```python
from build123d import *

# Parameters (mm, degrees)
SKETCH2_R          = 1.9177
CUT_EXTRUDE1_DEPTH = 33.764861657


with BuildPart() as part:
    # Sketch1 → Revolve1 (revolve)
    with BuildSketch(Plane.XY, mode=Mode.PRIVATE) as revolve1_sk:
        with BuildLine():
            Line((0, 0), (0, 30.1625))
            Line((0, 30.1625), (4.953, 30.1625))
            Line((4.953, 30.1625), (5.588, 20.76733075))
            Line((5.588, 20.76733075), (6.904482, 20.76733075))
            Line((6.904482, 20.76733075), (7.04215, 19.64973075))
            ThreePointArc((7.04215, 19.64973075), (4.64185, 17.316376969), (7.183974364, 15.1384))
            Line((7.183974364, 15.1384), (7.321642364, 14.0208))
            Line((7.321642364, 14.0208), (4.622892364, 14.0208))
            Line((4.622892364, 14.0208), (4.773075636, 12.8016))
            Line((4.773075636, 12.8016), (7.471825636, 12.8016))
            Line((7.471825636, 12.8016), (7.609493636, 11.684))
            Line((7.609493636, 11.684), (4.910743636, 11.684))
            Line((4.910743636, 11.684), (5.060926909, 10.4648))
            Line((5.060926909, 10.4648), (7.759676909, 10.4648))
            Line((7.759676909, 10.4648), (7.897344909, 9.3472))
            Line((7.897344909, 9.3472), (5.198594909, 9.3472))
            Line((5.198594909, 9.3472), (5.348778182, 8.128))
            Line((5.348778182, 8.128), (8.047528182, 8.128))
            Line((8.047528182, 8.128), (8.185196182, 7.0104))
            Line((8.185196182, 7.0104), (5.486446182, 7.0104))
            Line((5.486446182, 7.0104), (5.636629455, 5.7912))
            Line((5.636629455, 5.7912), (8.335379455, 5.7912))
            Line((8.335379455, 5.7912), (8.473047455, 4.6736))
            Line((8.473047455, 4.6736), (5.774297455, 4.6736))
            Line((5.774297455, 4.6736), (5.924480727, 3.4544))
            Line((5.924480727, 3.4544), (8.623230727, 3.4544))
            Line((8.623230727, 3.4544), (8.760898727, 2.3368))
            Line((8.760898727, 2.3368), (6.062148727, 2.3368))
            Line((6.062148727, 2.3368), (6.212332, 1.1176))
            Line((6.212332, 1.1176), (8.911082, 1.1176))
            Line((8.911082, 1.1176), (9.04875, 0))
            Line((9.04875, 0), (0, 0))
        make_face()
    revolve(revolve1_sk.sketch.rotate(Axis((0, 0, 0), (0, 1, 0)), 90), axis=Axis((0, 0, 0), (0, 1, 0)))

    # Sketch2 → Cut-Extrude1 (cut, through all)
    with BuildSketch(Plane(origin=(0, 30.1625, 0), x_dir=(1, 0, 0), z_dir=(0, 1, 0))):
        with Locations(Location((0, 0, 0), (0, 0, 270))):
            Circle(SKETCH2_R)
    extrude(amount=-CUT_EXTRUDE1_DEPTH, mode=Mode.SUBTRACT)


solid = part.part
```
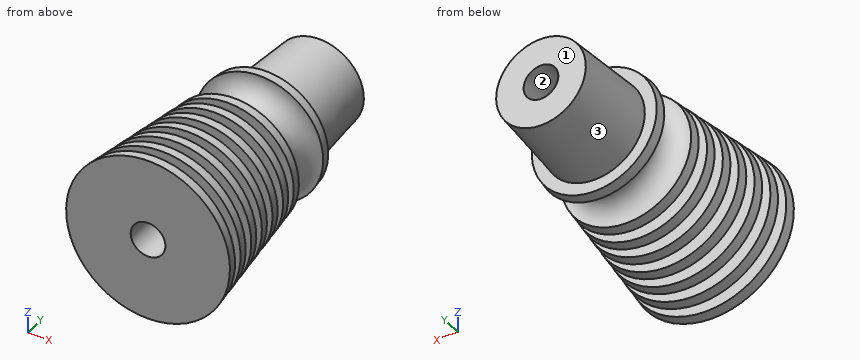
Design review of the part built by this model. Coordinates are the model's own, in mm. Face numbers are marked on the shaded views. Round coordinates to 2 decimals unless told otherwise and drop trailing zeros. Write each loop counter-clockwise with the first axis right and the second up, starting at its lowest first coordinate (ties: lowest second). Pieces come first, ordered by that corner, then holes.
Item 1: The part is to be moulded in two halves that separate along Z. For the marked faces 1, 2 and 3, say which applies: +Z half, -Z half, draft (parallel to the pull), parting line (faces both ways), or undercut.
Item 2: For probe 1 along X at (y, z) = (20.5, -1.75); probe 2 along X at (y, z) = (11, 0) (3 decimals); probe 3 along X at (y, z) = (9.5, 2.5), list the stretches that pass through material, from the lowest coordinate up.
Item 3: We need section A-A on y = 7.5. Write out the cut boundary in (x, z), and give its area (3 significant figures).
Item 4: Clearance check with flat-ended pins moving along their axes: pin 1 Ø3 at (x, z) = (-5, 1) entering from -Y; pin 2 Ø8 at (x, y) = (6.5, 13.5) entering from +Z; pin 3 Ø2.5 at (x, z) = (0, 0) entering from -Y; pin 4 Ø1 at (x, y) = (-2, 8.5) entering from -Z. State where each tip first meets the part, or that it passes through.
Returned:
1. face 1: draft
1. face 2: undercut
1. face 3: parting line
2. probe 1: x = -6.71 to -0.78, 0.78 to 6.71
2. probe 2: x = -4.995 to -1.918, 1.918 to 4.995
2. probe 3: x = -7.47 to 7.47
3. outline: circle Ø16.25 at (0, 0); hole circle Ø3.84 at (0, 0)
3. area: 196 mm2
4. pin 1: stops at y = 0
4. pin 2: stops at z = 7.04
4. pin 3: passes through
4. pin 4: stops at z = -7.87
